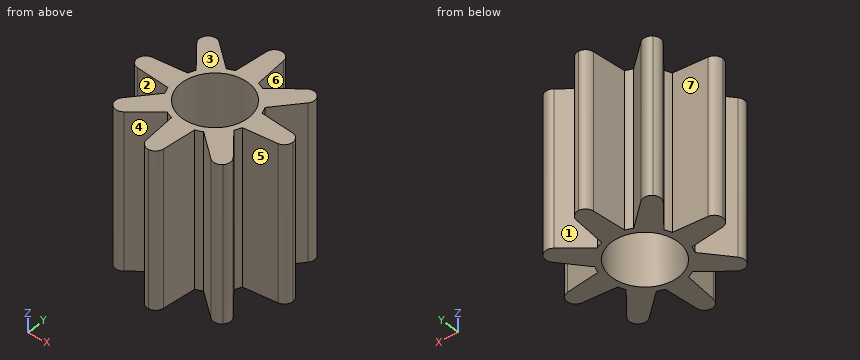
Autodesk Fusion 360 part; units mm, degrees
sketch "Small Head Gear" plane through (0, 0, 0) normal (0, 0, 1) x (1, 0, 0)
  circle A0 centre (0, 0) radius 1.0625
  arc A1 (-0.583, -1.1057) -> (-0.3696, -1.1941) centre (0, 0) ccw
  arc A2 (-1.1941, -0.3696) -> (-1.1057, -0.583) centre (0, 0) ccw
  arc A3 (-1.1057, 0.583) -> (-1.1941, 0.3696) centre (0, 0) ccw
  arc A4 (-0.3696, 1.1941) -> (-0.583, 1.1057) centre (0, 0) ccw
  arc A5 (0.583, 1.1057) -> (0.3696, 1.1941) centre (0, 0) ccw
  arc A6 (1.1941, 0.3696) -> (1.1057, 0.583) centre (0, 0) ccw
  arc A7 (0.3696, -1.1941) -> (0.583, -1.1057) centre (0, 0) ccw
  arc A8 (1.1057, -0.583) -> (1.1941, -0.3696) centre (0, 0) ccw
  line L0 (0, -2.5) -> (0.001, -2.5)
  line L1 (0, -2.5) -> (-0.001, -2.5)
  line L2 (1.7678, -1.7678) -> (1.7684, -1.7671)
  line L3 (1.7678, -1.7678) -> (1.7671, -1.7684)
  line L4 (1.7678, 1.7678) -> (1.7671, 1.7684)
  line L5 (1.7678, 1.7678) -> (1.7684, 1.7671)
  line L6 (0, 2.5) -> (-0.001, 2.5)
  line L7 (0, 2.5) -> (0.001, 2.5)
  line L8 (-1.7678, 1.7678) -> (-1.7684, 1.7671)
  line L9 (-1.7678, 1.7678) -> (-1.7671, 1.7684)
  line L10 (-2.5, 0) -> (-2.5, -0.001)
  line L11 (-2.5, 0) -> (-2.5, 0.001)
  line L12 (-1.7678, -1.7678) -> (-1.7671, -1.7684)
  line L13 (-1.7678, -1.7678) -> (-1.7684, -1.7671)
  line L14 (-0.3696, -1.1941) -> (-0.2729, -2.2501)
  line L15 (0.2729, -2.2501) -> (0.3696, -1.1941)
  line L16 (0.583, -1.1057) -> (1.3981, -1.784)
  line L17 (1.784, -1.3981) -> (1.1057, -0.583)
  line L18 (1.1941, -0.3696) -> (2.2501, -0.2729)
  line L19 (2.2501, 0.2729) -> (1.1941, 0.3696)
  line L20 (1.1057, 0.583) -> (1.784, 1.3981)
  line L21 (1.3981, 1.784) -> (0.583, 1.1057)
  line L22 (0.3696, 1.1941) -> (0.2729, 2.2501)
  line L23 (-0.2729, 2.2501) -> (-0.3696, 1.1941)
  line L24 (-0.583, 1.1057) -> (-1.3981, 1.784)
  line L25 (-1.784, 1.3981) -> (-1.1057, 0.583)
  line L26 (-1.1941, 0.3696) -> (-2.2501, 0.2729)
  line L27 (-2.2501, -0.2729) -> (-1.1941, -0.3696)
  line L28 (-1.1057, -0.583) -> (-1.784, -1.3981)
  line L29 (-1.3981, -1.784) -> (-0.583, -1.1057)
  line L30 (2.5, -0.001) -> (2.5, 0.001)
  arc A9 (-0.2729, -2.2501) -> (0.001, -2.5) centre (0.001, -2.225) ccw
  arc A10 (-0.001, -2.5) -> (0.2729, -2.2501) centre (-0.001, -2.225) ccw
  arc A11 (1.3981, -1.784) -> (1.7684, -1.7671) centre (1.574, -1.5726) ccw
  arc A12 (1.7671, -1.7684) -> (1.784, -1.3981) centre (1.5726, -1.574) ccw
  arc A13 (2.2501, -0.2729) -> (2.5, 0.001) centre (2.225, 0.001) ccw
  arc A14 (2.5, -0.001) -> (2.2501, 0.2729) centre (2.225, -0.001) ccw
  arc A15 (1.784, 1.3981) -> (1.7671, 1.7684) centre (1.5726, 1.574) ccw
  arc A16 (1.7684, 1.7671) -> (1.3981, 1.784) centre (1.574, 1.5726) ccw
  arc A17 (0.2729, 2.2501) -> (-0.001, 2.5) centre (-0.001, 2.225) ccw
  arc A18 (0.001, 2.5) -> (-0.2729, 2.2501) centre (0.001, 2.225) ccw
  arc A19 (-1.3981, 1.784) -> (-1.7684, 1.7671) centre (-1.574, 1.5726) ccw
  arc A20 (-1.7671, 1.7684) -> (-1.784, 1.3981) centre (-1.5726, 1.574) ccw
  arc A21 (-2.2501, 0.2729) -> (-2.5, -0.001) centre (-2.225, -0.001) ccw
  arc A22 (-2.5, 0.001) -> (-2.2501, -0.2729) centre (-2.225, 0.001) ccw
  arc A23 (-1.7684, -1.7671) -> (-1.3981, -1.784) centre (-1.574, -1.5726) ccw
  arc A24 (-1.784, -1.3981) -> (-1.7671, -1.7684) centre (-1.5726, -1.574) ccw
extrude "Extrude1" add sketch "Small Head Gear" along normal blind 5
Part model, mm, in its own coordinate system. Face numbers are marked on the shaded views. A direction names the side the tool comes from. Round coordinates to 2 decimals unless told otherwise and drop trailing zeros. Write each loop counter-clockwise with the first axis right and the second up, starting at its lowest first coordinate (ties: lowest second). Pieces come first, ordered by that corner, then holes. Notation, with made-up numbers: M 15,70 L 53,70 A15 cw 53,95 Z; hole C -33.5,49 d7. An arc over 180 degrees is marked long. One line per question, with ' | ' between items.
(1) 3-axis set-ups, long thin cutter, end or side, ignore diameter. For the marked faces 4, 5, 6 and 7: which of +Z, -Z, +X, -X, +Y, -Y reach the whole face in a straight line?
Answer key:
face 4: +Z, -Z, -Y | face 5: +Z, -Z, +X | face 6: +Z, -Z, +Y | face 7: +Z, -Z, -X
(2) Probe line 1 along Y through (x, z) = (0, 3.1); line 2 along X through (y, z) = (-1.25, 1.8). List the from-to ranges inside material, lowest first.
Answer key:
line 1: y = -2.5 to -1.06, 1.06 to 2.5 | line 2: x = -1.66 to -0.76, -0.36 to 0.36, 0.76 to 1.66
(3) Two-plate mould, pull along Y, no slides. Class the marked faces 1, 2 and 3: released by +Y, released by -Y, zero draft, split by the parting line, or undercut.
Answer key:
face 1: released by +Y | face 2: undercut | face 3: zero draft
(4) Pin check, flat tip, straight feed: pin 1 (3 mm diameter, centred on x = -2, z = 2.5, fed in from -Y). Stop position of the tip, or through.
Answer key:
pin 1: stops at y = -1.85
(5) Saw through at A-A on x = -0.15. Write the cut outline in (y, z), then the cut area to 3 significant figures.
Answer key:
outline: M -2.45,0 L -1.05,0 L -1.05,5 L -2.45,5 Z; M 1.05,0 L 2.45,0 L 2.45,5 L 1.05,5 Z | area: 14.0 mm^2
(6) Saw through at B-B on y = 0.7. Write the cut outline in (x, z), then the cut area to 3 significant figures.
Answer key:
outline: M -1.2,0 L -0.8,0 L -0.8,5 L -1.2,5 Z; M 0.8,0 L 1.2,0 L 1.2,5 L 0.8,5 Z | area: 4.04 mm^2
(7) Saw through at D-D on x = 2. Write the cut outline in (y, z).
Answer key:
outline: M -0.3,0 L 0.3,0 L 0.3,5 L -0.3,5 Z
(8) Saw through at C-C on y = 1.65. Write the cut outline in (x, z).
Answer key:
outline: M -1.84,0 L -1.24,0 L -1.24,5 L -1.84,5 Z; M -0.33,0 L 0.33,0 L 0.33,5 L -0.33,5 Z; M 1.24,0 L 1.84,0 L 1.84,5 L 1.24,5 Z
